```python
from build123d import *
from OCP.BRepAlgoAPI import BRepAlgoAPI_Cut
from OCP.TopTools import TopTools_ListOfShape

# Parameters (mm, degrees)
SKETCH10_R              = 1.5
BOSS_EXTRUDE2_DEPTH     = 18
CUT_EXTRUDE1_DEPTH      = 53
CUT_EXTRUDE1_DEPTH_BACK = 21
SKETCH12_R              = 101.363268326
CUT_EXTRUDE2_DEPTH      = 4
CUT_EXTRUDE3_DEPTH      = 4
CUT_EXTRUDE3_DEPTH_BACK = 4
CUT_EXTRUDE4_DEPTH      = 149.963082804
CUT_EXTRUDE4_DEPTH_BACK = 149.963082804
CUT_EXTRUDE5_DEPTH      = 123.927520285
CUT_EXTRUDE5_DEPTH_BACK = 123.927520285


with BuildPart() as part:
    # Sketch10 → Boss-Extrude2 (new body)
    with BuildSketch(Plane.XY):
        with BuildLine():
            Line((37.416573868, 15), (102.583426132, 15))
            ThreePointArc((102.583426132, 15), (121.439606964, 10.276684148), (135.842602904, -2.777777778))
            ThreePointArc((135.842602904, -2.777777778), (142.889960635, -4.080211701), (144, 3))
            ThreePointArc((144, 3), (124.596747752, 19.193495505), (100, 25))
            Line((100, 25), (40, 25))
            ThreePointArc((40, 25), (15.403252248, 19.193495505), (-4, 3))
            ThreePointArc((-4, 3), (-2.889960635, -4.080211701), (4.157397096, -2.777777778))
            ThreePointArc((4.157397096, -2.777777778), (18.560393036, 10.276684148), (37.416573868, 15))
        make_face()
        Circle(SKETCH10_R, mode=Mode.SUBTRACT)
        with Locations(Location((140, 0, 0), (0, 0, 180))):
            Circle(SKETCH10_R, mode=Mode.SUBTRACT)
    extrude(amount=BOSS_EXTRUDE2_DEPTH)

    # Sketch12 → Cut-Extrude1 (cut, two sides: drawn at the far end of the back side and taken through both)
    with BuildSketch(Plane(origin=(0, 0, 0), x_dir=(1, 0, 0), z_dir=(0, 1, 0)).offset(-CUT_EXTRUDE1_DEPTH_BACK)):
        with Locations((76.008049748, -10.931288324)):
            Circle(SKETCH12_R)
        with BuildLine():
            Line((-5, -6), (-5, -14))
            Line((-5, -14), (107.805696866, -14))
            ThreePointArc((107.805696866, -14), (113.026744555, -14.342205545), (118.15845867, -15.362966948))
            Line((118.15845867, -15.362966948), (122.913338099, -16.637033052))
            ThreePointArc((122.913338099, -16.637033052), (128.045052215, -17.657794455), (133.266099903, -18))
            Line((133.266099903, -18), (145, -18))
            Line((145, -18), (145, -14))
            Line((145, -14), (130, -14))
            Line((130, -14), (126.989127027, -13.193239018))
            ThreePointArc((126.989127027, -13.193239018), (125.143296129, -10.589859532), (127.359731004, -8.293755679))
            Line((127.359731004, -8.293755679), (130, -8))
            Line((130, -8), (145, -8))
            Line((145, -8), (145, -4))
            Line((145, -4), (130.2183511, -4))
            ThreePointArc((130.2183511, -4), (128.003403615, -4.061371986), (125.795252917, -4.245299618))
            Line((125.795252917, -4.245299618), (112.228795048, -5.754700382))
            ThreePointArc((112.228795048, -5.754700382), (110.02064435, -5.938628014), (107.805696866, -6))
            Line((107.805696866, -6), (-5, -6))
        make_face(mode=Mode.SUBTRACT)
    extrude(amount=CUT_EXTRUDE1_DEPTH + CUT_EXTRUDE1_DEPTH_BACK, mode=Mode.SUBTRACT)


with BuildPart() as cut_extrude2_tool:
    # Sketch14 → Cut-Extrude2 (new body)
    with BuildSketch(Plane(origin=(0, 0, 6), x_dir=(-1, 0, 0), z_dir=(0, 0, -1))):
        with BuildLine():
            Line((-102.583426132, 16), (-37.416573868, 16))
            ThreePointArc((-37.416573868, 16), (-22.580527687, 13.221613437), (-9.75522645, 5.2630114))
            Line((-9.75522645, 5.2630114), (-4.407881121, 10.610356729))
            ThreePointArc((-4.407881121, 10.610356729), (-20.986311028, 20.541860192), (-40, 24))
            Line((-40, 24), (-100, 24))
            ThreePointArc((-100, 24), (-103.919892318, 23.857538416), (-107.819101893, 23.430905341))
            Line((-107.819101893, 23.430905341), (-107.819101893, 35.168317198))
            Line((-107.819101893, 35.168317198), (17.162371348, 35.168317198))
            Line((17.162371348, 35.168317198), (17.162371348, -18.766284645))
            Line((17.162371348, -18.766284645), (-107.819101893, -18.766284645))
            Line((-107.819101893, -18.766284645), (-107.819101893, 15.664329569))
            ThreePointArc((-107.819101893, 15.664329569), (-105.206638634, 15.915996336), (-102.583426132, 16))
        make_face()
    extrude(amount=-CUT_EXTRUDE2_DEPTH)


with BuildPart() as part_1:
    add(part.part)

    # Cut-Extrude2: cut by cut_extrude2_tool, with a tolerance
    cut_extrude2_stock = TopTools_ListOfShape()
    cut_extrude2_stock.Append(part_1.part.wrapped)
    cut_extrude2_tools = TopTools_ListOfShape()
    cut_extrude2_tools.Append(cut_extrude2_tool.part.wrapped)
    cut_extrude2_cut = BRepAlgoAPI_Cut()
    cut_extrude2_cut.SetArguments(cut_extrude2_stock)
    cut_extrude2_cut.SetTools(cut_extrude2_tools)
    cut_extrude2_cut.SetFuzzyValue(0.00001)
    cut_extrude2_cut.Build()
    add(Compound.cast(cut_extrude2_cut.Shape()).solids(), mode=Mode.REPLACE)

    # Sketch15 → Cut-Extrude3 (cut, two sides: drawn at the far end of the back side and taken through both)
    with BuildSketch(Plane(origin=(2.00470116, 0, 18.018205945), x_dir=(-0.9938675095528059, 0, 0.11057745455246941), z_dir=(-0.11057745455246942, 0, -0.993867509552806)).offset(-CUT_EXTRUDE3_DEPTH_BACK)):
        with BuildLine():
            Line((-119.163095282, 20.093526394), (-118.740012656, 11.822126877))
            add(Edge.make_bspline(
                [(-118.740012656, 11.822126877), (-114.62508956, 13.623450352), (-110.296692622, 14.978589212), (-105.908841603, 15.833395956)],
                knots=[-1.219718725, -1.219718725, -1.219718725, -1.219718725, -0.997934063, -0.997934063, -0.997934063, -0.997934063], degree=3))
            Line((-105.908841603, 15.833395956), (-105.908841603, 7.414190779))
            Line((-105.908841603, 7.414190779), (-142.752233985, -17.524399772))
            Line((-142.752233985, -17.524399772), (-150.166718445, 16.856471942))
            Line((-150.166718445, 16.856471942), (-106.447848094, 34.09271449))
            Line((-106.447848094, 34.09271449), (-105.908841603, 23.554966644))
            add(Edge.make_bspline(
                [(-105.908841603, 23.554966644), (-110.40344818, 22.781977164), (-114.85327417, 21.619160072), (-119.163095282, 20.093526394)],
                knots=[-1.323472262, -1.323472262, -1.323472262, -1.323472262, -1.152490077, -1.152490077, -1.152490077, -1.152490077], degree=3))
        make_face()
    extrude(amount=CUT_EXTRUDE3_DEPTH + CUT_EXTRUDE3_DEPTH_BACK, mode=Mode.SUBTRACT)

    # Sketch16 → Cut-Extrude4 (cut, two sides: drawn at the far end of the back side and taken through both)
    with BuildSketch(Plane(origin=(0, 24, 0), x_dir=(1, 0, 0), z_dir=(0, 1, 0)).offset(-CUT_EXTRUDE4_DEPTH_BACK)):
        Polygon((3.407881121, -7), (109.942912406, -7), (121.047014556, -5.863668195), (121.047014556, -0.454097239), (147.279060568, 4.078614092), (150.076867714, -41.016929059), (122.104873778, -29.787827075), (117.671018844, -29.787827075), (117.671018844, -30.883133113), (3.407881121, -30.883133113), (-7.729647631, -28.692521036), (-16.239396681, -3.124111032), (3.407881121, -0.69185953), align=None)
    extrude(amount=CUT_EXTRUDE4_DEPTH + CUT_EXTRUDE4_DEPTH_BACK, mode=Mode.SUBTRACT)

    # Sketch17 → Cut-Extrude5 (cut, two sides: drawn at the far end of the back side and taken through both)
    with BuildSketch(Plane(origin=(0, 0, 6), x_dir=(-1, 0, 0), z_dir=(0, 0, -1)).offset(-CUT_EXTRUDE5_DEPTH_BACK)):
        Polygon((-4.33267462, 12.099776793), (-11.665353096, 4.767098316), (-11.583019887, 4.684765107), (-10.593616865, 3.695362084), (-1.134184227, 10.251312954), align=None)
        Polygon((-119.713110979, 21.610434881), (-119.111195403, 9.770184261), (-121.889059026, 7.660492949), (-122.569179785, 21.039113751), align=None)
    extrude(amount=CUT_EXTRUDE5_DEPTH + CUT_EXTRUDE5_DEPTH_BACK, mode=Mode.SUBTRACT)


solid = part_1.part
```
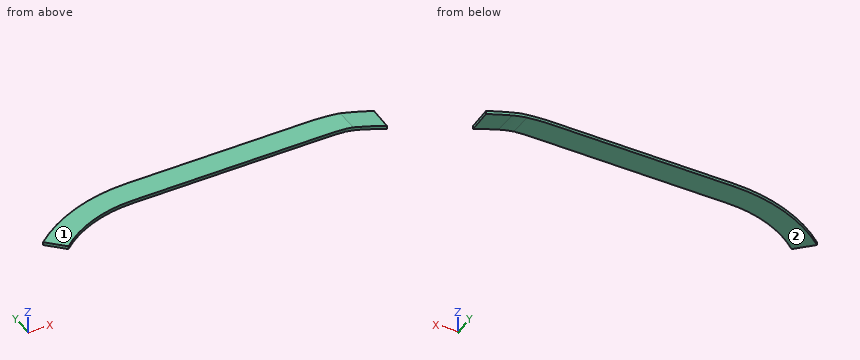
Check sheet for the modelled part. Datum: model origin and axes. Units: mm. Face numbers are marked on the shaded views. A direction names the side the tool comes from. Round coordinates to 2 decimals unless told otherwise and drop trailing zeros. Loops run counter-clockwise (first coordinate to the right, second up) from the corner with the lowest first, then second, coordinate; pieces in that order, holes last. Notation, with made-up numbers: (-10, 66.25) -> (22, 66.25) arc R30 ccw to (22, 94.25) -> close; hole circle Ø2 at (-4, 87.25). An arc over 180 degrees is marked (long way). Answer in a Markdown table with one row per item.
Q1. Sectioned sample at C-C on x = 33.5. Enter the section's corners in (y, z), then the cut area to 3 significant figures.
Data:
| item | result |
|---|---|
| outline | (15.81, 6) -> (23.61, 6) -> (23.61, 7) -> (15.81, 7) -> close |
| area | 7.79 mm^2 |
Q2. Go/stop test with flat-tipped pins: P1, Ø0.8, axis at x = 66.5, z = 6.5, coming from the -Y side; P2, Ø5, axis at x = 80, y = 19.5, coming from the -Z side; P3, Ø5, axis at x = 104, y = 13, coming from the +Z side. Record where each tip stops, or that it passes through.
Data:
| item | result |
|---|---|
| P1 | stops at y = 16 |
| P2 | stops at z = 6 |
| P3 | passes through |
Q3. Set-up check for the marked faces 1 and 2: record each of +Z, -Z, +X, -X, +Y, -Y from which the full face is reachable in a straight line by a thin tool's end or side.
Data:
| item | result |
|---|---|
| face 1 | +Z, +X, -X, +Y, -Y |
| face 2 | -Z, -X, +Y, -Y |
Q4. Sectioned sample at B-B on x = 88. Enter the section's corners in (y, z), then the cut area to 3 significant figures.
Data:
| item | result |
|---|---|
| outline | (16, 6) -> (24, 6) -> (24, 7) -> (16, 7) -> close |
| area | 8.00 mm^2 |
Q5. Sectioned sample at A-A on y = 18.75. Enter the section's corners in (x, z), then the cut area to 3 significant figures.
Data:
| item | result |
|---|---|
| outline | (16.77, 6) -> (107.81, 6) arc R40 cw to (112.23, 5.75) -> (119.57, 4.94) -> (119.57, 6.02) -> (109.94, 7) -> (16.77, 7) -> close |
| area | 103 mm^2 |
Q6. Thickness scan on L1, parallel to Z at x = 75.5, y = 17.75; L2, parallel to Y at x = 74.5, z = 6.55; L3, parallel to X at y = 12.75, z = 6.7. Record the ranges inside material, lowest first.
Data:
| item | result |
|---|---|
| L1 | z = 6 to 7 |
| L2 | y = 16 to 24 |
| L3 | x = 7.01 to 21.42 |
